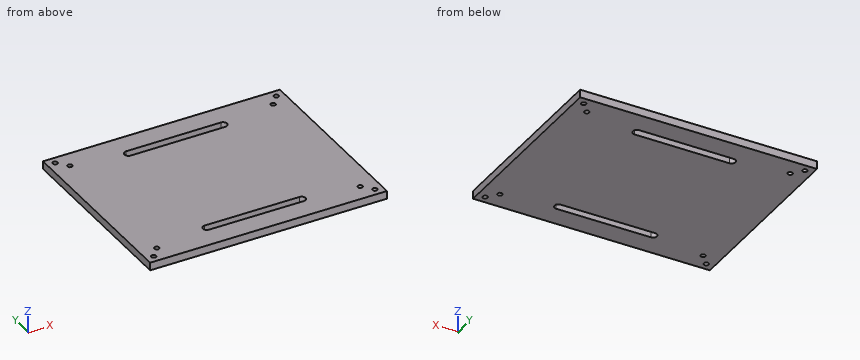
from build123d import *

# Parameters (mm, degrees)
MODEL_W             = 150
MODEL_H             = 120
MODEL_R             = 1.5
BOSS_EXTRUDE1_DEPTH = 5
CUT_EXTRUDE1_DEPTH  = 209.993753976


with BuildPart() as part:
    # Model → Boss-Extrude1 (new body)
    with BuildSketch(Plane.XY):
        with Locations((88.925313808, 69.54489837)):
            Rectangle(MODEL_W, MODEL_H)
        with Locations((18.879939798, 124.771335066)):
            Circle(MODEL_R, mode=Mode.SUBTRACT)
        with Locations((158.970687817, 124.771335066)):
            Circle(MODEL_R, mode=Mode.SUBTRACT)
        with Locations((18.879939798, 14.318461674)):
            Circle(MODEL_R, mode=Mode.SUBTRACT)
        with Locations((158.970687817, 14.318461674)):
            Circle(MODEL_R, mode=Mode.SUBTRACT)
        with Locations((24.548687541, 118.224668434)):
            Circle(MODEL_R, mode=Mode.SUBTRACT)
        with Locations((153.301940075, 118.224668434)):
            Circle(MODEL_R, mode=Mode.SUBTRACT)
        with Locations((24.548687541, 20.865128307)):
            Circle(MODEL_R, mode=Mode.SUBTRACT)
        with Locations((153.301940075, 20.865128307)):
            Circle(MODEL_R, mode=Mode.SUBTRACT)
    extrude(amount=BOSS_EXTRUDE1_DEPTH)

    # Sketch2 → Cut-Extrude1 (cut, through all)
    with BuildSketch(Plane(origin=(0, 0, 0), x_dir=(-1, 0, 0), z_dir=(0, 0, -1))):
        with BuildLine():
            Line((-58.929782285, 110.90640838), (-118.938578053, 111.011957594))
            ThreePointArc((-118.938578053, 111.011957594), (-121.474611242, 113.556927738), (-118.929641098, 116.092960927))
            Line((-118.929641098, 116.092960927), (-58.92084533, 115.987411713))
            ThreePointArc((-58.92084533, 115.987411713), (-56.384812141, 113.442441569), (-58.929782285, 110.90640838))
        make_face()
        with BuildLine():
            Line((-58.921024216, 23.204088411), (-118.929819984, 23.098539197))
            ThreePointArc((-118.929819984, 23.098539197), (-121.372907859, 25.533047888), (-118.938399168, 27.976135764))
            Line((-118.938399168, 27.976135764), (-58.9296034, 28.081684978))
            ThreePointArc((-58.9296034, 28.081684978), (-56.486515525, 25.647176286), (-58.921024216, 23.204088411))
        make_face()
    extrude(amount=-CUT_EXTRUDE1_DEPTH, mode=Mode.SUBTRACT)


solid = part.part
Source: CAD feature listing. Evaluate the final solid. Frame: model axes, mm. Give positions to 0.01 mm unless a question says otherwise; leave off trailing zeros. Write each loop counter-clockwise with the first axis right and the second up, starting at its lowest first coordinate (ties: lowest second). Pieces come first, ordered by that corner, then holes. Notation, with made-up numbers: M 56,65 L 73,65 A35 cw 73,98 Z; hole C -6.5,78.25 d10. An arc over 180 degrees is marked long. Return JSON: item names as keys, results as strings. Group by question number.
1) Material intervals for line 1 along Y through (x, z) = (72.5, 1.2); line 2 along Y through (x, z) = (103, 1.2); line 3 along X through (y, z) = (24.5, 1.3), sorted ascending. Write a range as [from, to].
2) Pin query (flat end, axial travel): P1, Ø2.5, axis at x = 153.3, y = 118.22, coming from the +Z side; P2, Ø4, axis at x = 18.88, y = 14.32, coming from the +Z side. Return the tip coordinate at first contact, or that it passes through.
3) Cut plane C-C, the plane y = 26. Output: boundary loops of the cut face in (x, z), plus the area to 3 significant figures.
4) Cut plane A-A, the plane x = 111.5. Output: boundary loops of the cut face in (y, z), plus the area to 3 significant figures.
5) Cut plane B-B, the plane z = 1.6. Give the number of separate pieces and of enclosed holes in the cut face, plus the area to 3 significant figures.
Recorded:
{
 "1": {"line 1": "y = [9.54, 23.18], [28.06, 110.93], [116.01, 129.54]", "line 2": "y = [9.54, 23.13], [28, 110.98], [116.06, 129.54]", "line 3": "x = [13.93, 56.77], [121.14, 163.93]"},
 "2": {"P1": "passes through", "P2": "stops at z = 5"},
 "3": {"outline": "M 13.93,0 L 56.51,0 L 56.51,5 L 13.93,5 Z; M 121.33,0 L 163.93,0 L 163.93,5 L 121.33,5 Z", "area": "426 mm²"},
 "4": {"outline": "M 9.54,0 L 23.11,0 L 23.11,5 L 9.54,5 Z; M 27.99,0 L 111,0 L 111,5 L 27.99,5 Z; M 116.08,0 L 129.54,0 L 129.54,5 L 116.08,5 Z", "area": "550 mm²"},
 "5": {"separate pieces": "1", "enclosed holes": "10", "area": "17,300 mm²"}
}
